CAD build for the part. Positions are in the model's coordinates, mm. A direction names the side the tool comes from. Round coordinates to 2 decimals unless told otherwise and drop trailing zeros. Write each loop counter-clockwise with the first axis right and the second up, starting at its lowest first coordinate (ties: lowest second). Pieces come first, ordered by that corner, then holes. Notation, with made-up numbers: (27, -19.75) -> (32, -19.75) arc R15 ccw to (32, -15.75) -> close; hole circle Ø11 at (44, -1). An arc over 180 degrees is marked (long way). Put each result on its own line as item: value. Start each with the question number.
1. 3-axis set-ups, long thin cutter, end or side, ignore diameter. For faces 5 (the flat face through (71.12, 2, -1)), 6 (the flat face through (64.77, -1, -40)), 7 (the flat face through (58, 3, -30.257)): which of +Z, -Z, +X, -X, +Y, -Y reach the whole face in a straight line?
2. Flat gauge pins, fed straight in: P1, Ø6, axis at x = 22.5, z = -26, coming from the -Y side; P2, Ø5, axis at y = 2.5, z = -20, coming from the +X side. Where does each tip first touch, or does it go through?
3. Drill centre lines: line 1 (Z direction, x = 31, y = -0.25); line 2 (X direction, y = 1.5, z = -2.54); line 3 (Z direction, x = 51.5, y = 4). Where is each one in solid material? Low to high. Write a range as from..to.
4. Saw through at B-B on z = -2.54. List the corners of the cut face in (x, y), and give its area (3 significant figures).
5. Saw through at D-D on z = -39.5. List the corners of the cut face in (x, y), and give its area (3 significant figures).
6. Saw through at C-C on x = 59.69. List the corners of the cut face in (y, z), and give its area (3 significant figures).
7. Pull direction X, two halves, no side cores. Call faces 1 (the flat face through (32, -1, -50.8)), 2 (the cylindrical face through (-5.626, 1.843, -57.531)), 3 (the cylindrical face through (70.356, 1.967, 4.481)), 4 (the flat face through (32, 6.35, -27)): pulls with the +X half, pulls with the -X half, needs draft (parallel to the pull), parting line crosses it, or undercut.
8. Saw through at A-A on x = 8.89. List the corners of the cut face in (y, z), and give its area (3 significant figures).
from build123d import *

# Parameters (mm, degrees)
SKETCH1_W           = 77.47
SKETCH1_H           = 63.5
SKETCH1_W_2         = 64.77
SKETCH1_H_2         = 50.8
BOSS_EXTRUDE1_DEPTH = 6.35
SKETCH1_3_W         = 77.47
SKETCH1_3_H         = 63.5
SKETCH1_3_W_2       = 64.77
SKETCH1_3_H_2       = 50.8
BOSS_EXTRUDE2_DEPTH = 2.54
SKETCH2_W           = 25.4
SKETCH2_H           = 25.4
CUT_EXTRUDE1_DEPTH  = 12.7
SKETCH3_R           = 2.1
CUT_EXTRUDE2_DEPTH  = 12.7
FILLET1_R           = 2.54
SKETCH4_R           = 1.5
CUT_EXTRUDE3_DEPTH  = 22.86


with BuildPart() as part:
    # Sketch1 → Boss-Extrude1 (new body)
    # profile 1 of 2: a face of its own
    with BuildSketch(Plane(origin=(0, 0, 0), x_dir=(1, 0, 0), z_dir=(0, 1, 0))):
        with Locations((32.385, 26.545081967)):
            Rectangle(SKETCH1_W, SKETCH1_H)
        with Locations((32.385, 25.4)):
            Rectangle(SKETCH1_W_2, SKETCH1_H_2, mode=Mode.SUBTRACT)
    # profile 2 of 2: a face of its own
    with BuildSketch(Plane(origin=(0, 0, 0), x_dir=(1, 0, 0), z_dir=(0, 1, 0))):
        with Locations((32.385, 25.4)):
            Rectangle(SKETCH1_W_2, SKETCH1_H_2)
    extrude(amount=BOSS_EXTRUDE1_DEPTH)

    # Sketch1_3 → Boss-Extrude2 (add)
    with BuildSketch(Plane(origin=(0, 0, 0), x_dir=(1, 0, 0), z_dir=(0, 1, 0))):
        with Locations((32.385, 26.545081967)):
            Rectangle(SKETCH1_3_W, SKETCH1_3_H)
        with Locations((32.385, 25.4)):
            Rectangle(SKETCH1_3_W_2, SKETCH1_3_H_2, mode=Mode.SUBTRACT)
    extrude(amount=-BOSS_EXTRUDE2_DEPTH)

    # Sketch2 → Cut-Extrude1 (cut)
    with BuildSketch(Plane.XZ.offset(2.54)):
        with Locations((58.42, -17.556565957)):
            Rectangle(SKETCH2_W, SKETCH2_H)
    extrude(amount=-CUT_EXTRUDE1_DEPTH, mode=Mode.SUBTRACT)

    # Sketch3 → Cut-Extrude2 (cut)
    with BuildSketch(Plane.XZ.offset(2.54)):
        with Locations(Location((-3.175, 2.029918033, 0), (0, 0, 270))):
            Circle(SKETCH3_R)
        with Locations(Location((-3.175, -55.120081967, 0), (0, 0, 270))):
            Circle(SKETCH3_R)
        with Locations(Location((67.945, -55.120081967, 0), (0, 0, 270))):
            Circle(SKETCH3_R)
    extrude(amount=-CUT_EXTRUDE2_DEPTH, mode=Mode.SUBTRACT)

    # Fillet1
    fillet1_edges = [part.edges().sort_by_distance(p)[0] for p in [
        (71.12, 1.905, -58.295081967),
        (71.12, 1.905, 5.204918033),
        (-6.35, 1.905, 5.204918033),
        (-6.35, 1.905, -58.295081967),
    ]]
    fillet(fillet1_edges, radius=FILLET1_R)

    # Sketch4 → Cut-Extrude3 (cut)
    with BuildSketch(Plane.XZ):
        with Locations(Location((59.69, -2.54, 0), (0, 0, 270))):
            Circle(SKETCH4_R)
        with Locations(Location((8.89, -2.54, 0), (0, 0, 270))):
            Circle(SKETCH4_R)
    extrude(amount=-CUT_EXTRUDE3_DEPTH, mode=Mode.SUBTRACT)


solid = part.part
Return value:
1. face 5: +Z, -Z, +X, +Y, -Y
1. face 6: -Y
1. face 7: +X, +Y, -Y
2. P1: stops at y = 0
2. P2: stops at x = 45.72
3. line 1: z = -58.3..-50.8, 0..5.2
3. line 2: x = -6.35..7.39, 10.39..58.19, 61.19..71.12
3. line 3: z = -58.3..-30.26, -4.86..5.2
4. outline: (-6.35, -2.54) -> (0, -2.54) -> (0, 0) -> (7.39, 0) -> (7.39, 6.35) -> (-6.35, 6.35) -> close; (10.39, 0) -> (58.19, 0) -> (58.19, 6.35) -> (10.39, 6.35) -> close; (61.19, 0) -> (64.77, 0) -> (64.77, -2.54) -> (71.12, -2.54) -> (71.12, 6.35) -> (61.19, 6.35) -> close
4. area: 486 mm^2
5. outline: (-6.35, -2.54) -> (0, -2.54) -> (0, 0) -> (64.77, 0) -> (64.77, -2.54) -> (71.12, -2.54) -> (71.12, 6.35) -> (-6.35, 6.35) -> close
5. area: 524 mm^2
6. outline: (-2.54, -58.3) -> (6.35, -58.3) -> (6.35, -30.26) -> (0, -30.26) -> (0, -50.8) -> (-2.54, -50.8) -> close; (-2.54, 0) -> (0, 0) -> (0, -1.04) -> (6.35, -1.04) -> (6.35, 5.2) -> (-2.54, 5.2) -> close; (0, -4.86) -> (6.35, -4.86) -> (6.35, -4.04) -> (0, -4.04) -> close
6. area: 255 mm^2
7. face 1: undercut
7. face 2: pulls with the -X half
7. face 3: pulls with the +X half
7. face 4: needs draft
8. outline: (-2.54, -58.3) -> (6.35, -58.3) -> (6.35, -4.04) -> (0, -4.04) -> (0, -50.8) -> (-2.54, -50.8) -> close; (-2.54, 0) -> (0, 0) -> (0, -1.04) -> (6.35, -1.04) -> (6.35, 5.2) -> (-2.54, 5.2) -> close
8. area: 416 mm^2
